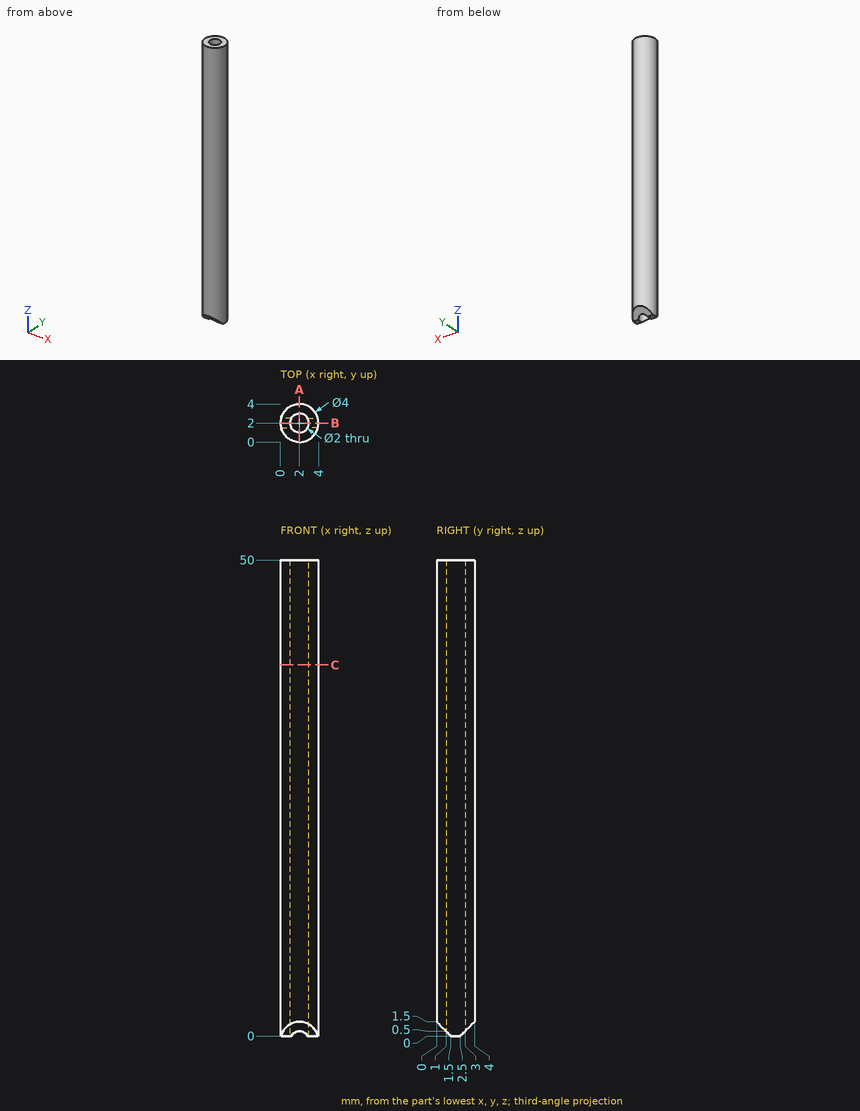
Design review of the part shown in the three views and the two pictorial views. Dimensions are in mm from the part's minimum x, y and z. Give positions to 0.01 mm unless a question says otherwise; leave off trailing zeros. Write each loop counter-clockwise with the first axis right and the second up, starting at its lowest first coordinate (ties: lowest second). Pieces come first, ordered by that corner, then holes. Notation, with made-up numbers: M 39.25,59.25 L 50.25,59.25 A19 ccw 50.25,92.25 Z; hole C 6,34.25 d6. An arc over 180 degrees is marked long. One line per item, written item: value.
1) Take a section at C-C, the plane z = 39. Write out the cut boundary in (x, y), then the cut area to 3 significant figures.
Results are:
outline: C 2,2 d4; hole C 2,2 d2
area: 9.42 mm²
2) Take a section at B-B, the plane y = 2. Write out the cut boundary in (x, z).
Results are:
outline: M 0,0 L 1,0 L 1,50 L 0,50 Z; M 3,0 L 4,0 L 4,50 L 3,50 Z
3) Take a section at A-A, the plane x = 2. Write out the cut boundary in (y, z), then the cut area to 3 significant figures.
Results are:
outline: M 0,1.5 L 1,0.5 L 1,50 L 0,50 Z; M 3,0.5 L 4,1.5 L 4,50 L 3,50 Z
area: 98.0 mm²
4) For P1, Ø1, axis at y = 3.5, z = 35.5, coming from the +X side, flat-tipped, find the tip position at first contact; note if it passes through.
Results are:
P1: stops at x = 3.73
5) For line 1 (X direction, y = 2, z = 12); line 2 (X direction, y = 1.5, z = 39.5), list the stretches that pass through material, from the lowest coordinate up. Write a range as from..to.
Results are:
line 1: x = 0..1, 3..4
line 2: x = 0.06..1.13, 2.87..3.94
